Source: three-view drawing plus pictorial views. Frame: mm from the lowest corner of the part. A direction names the side the tool comes from. Give positions to 0.01 mm unless a question says otherwise; leave off trailing zeros. Order: outer loops, then holes, each group sorted by start corner. A loop starts at its lowest first (then second) coordinate and runs counter-clockwise, first axis right, second up. Notation, with made-up numbers: (-27.75, 20) -> (25.25, 20) arc R23 ccw to (25.25, 33) -> close; hole circle Ø5 at (37.25, 57.25). An arc over 180 degrees is marked (long way). Answer in a Markdown table with one row per item.
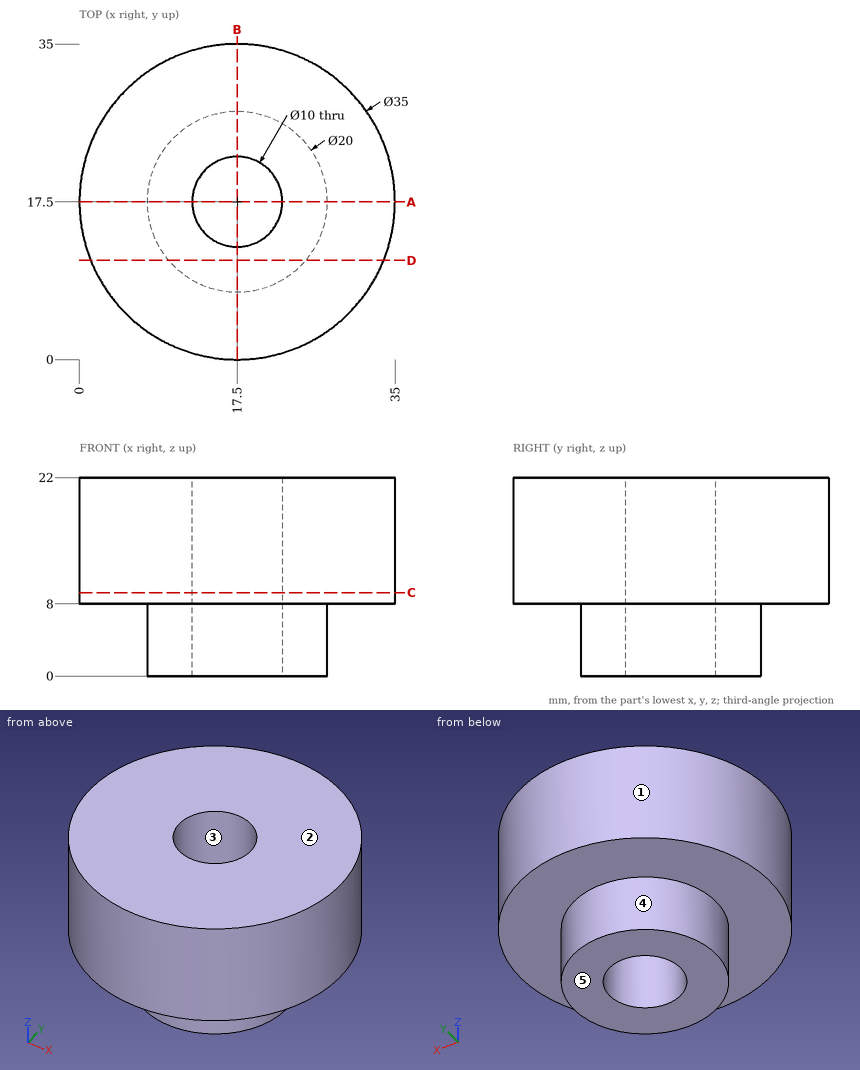
(1) Section query C-C (z = 9.25). Return the cut outline in (x, y), plus the area to 3 significant figures.
A:
| item | result |
|---|---|
| outline | circle Ø35 at (17.5, 17.5); hole circle Ø10 at (17.5, 17.5) |
| area | 884 mm^2 |
(2) Pull-direction query (Y, two-part tool) for the marked faces 1, 2 and 3; classes: +Y half, -Y half, draft (parallel to the pull), parting line (faces both ways), or undercut.
A:
| item | result |
|---|---|
| face 1 | parting line |
| face 2 | draft |
| face 3 | undercut |
(3) Ray query, probe 1 along Y at (x, z) = (17.5, 7.5); probe 2 along Z at (x, y) = (27.5, 8); probe 3 along Y at (x, z) = (20.5, 14.5). Return the intervals inside material, ascending.
A:
| item | result |
|---|---|
| probe 1 | y = 7.5 to 12.5, 22.5 to 27.5 |
| probe 2 | z = 8 to 22 |
| probe 3 | y = 0.26 to 13.5, 21.5 to 34.74 |
(4) Section query D-D (y = 11). Return the cut outline in (x, z), plus the area to 3 significant figures.
A:
| item | result |
|---|---|
| outline | (1.25, 8) -> (9.9, 8) -> (9.9, 0) -> (25.1, 0) -> (25.1, 8) -> (33.75, 8) -> (33.75, 22) -> (1.25, 22) -> close |
| area | 577 mm^2 |
(5) First-contact query: pin 1 Ø2 at (x, y) = (28.5, 16) entering from -Z; pin 2 Ø4 at (y, z) = (6.5, 19.5) entering from -X; pin 3 Ø6 at (y, z) = (6.5, 13) entering from +X; pin 4 Ø9 at (x, y) = (17.5, 17.5) entering from +Z. Flat tips, straight axial feed; report the tip coordinate or a pass-through.
A:
| item | result |
|---|---|
| pin 1 | stops at z = 8 |
| pin 2 | stops at x = 2.49 |
| pin 3 | stops at x = 33.06 |
| pin 4 | passes through |
(6) Access query for the marked faces 4 and 5. Directions: +Z, -Z, +X, -X, +Y, -Y. A direction counts if a zero-diameter tool reaches every point of the face in a straight line with its end or side. Return the directions, or none.
A:
| item | result |
|---|---|
| face 4 | -Z |
| face 5 | -Z, +X, -X, +Y, -Y |
(7) Section query A-A (y = 17.5). Return the cut outline in (x, z), plus the area to 3 significant figures.
A:
| item | result |
|---|---|
| outline | (0, 8) -> (7.5, 8) -> (7.5, 0) -> (12.5, 0) -> (12.5, 22) -> (0, 22) -> close; (22.5, 0) -> (27.5, 0) -> (27.5, 8) -> (35, 8) -> (35, 22) -> (22.5, 22) -> close |
| area | 430 mm^2 |
